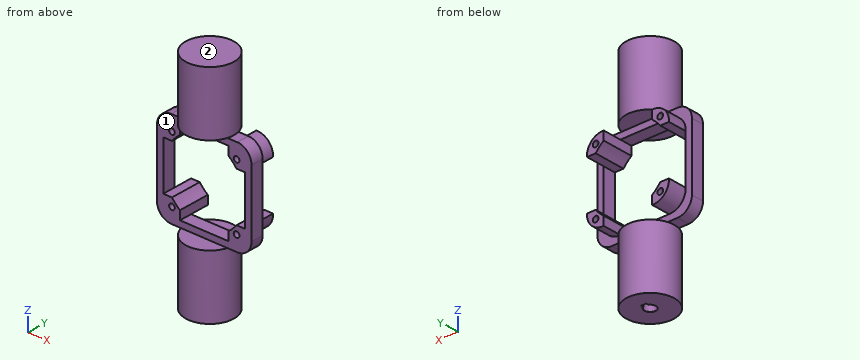
Autodesk Inventor part; units mm, degrees
ref_plane "YZ Plane" through (0, 0, 0) normal (1, 0, 0) x (0, 1, 0)
ref_plane "XZ Plane" through (0, 0, 0) normal (0, 1, 0) x (-1, 0, 0)
ref_plane "XY Plane" through (0, 0, 0) normal (0, 0, 1) x (1, 0, 0)
sketch "Sketch1" plane through (0, 0, 0) normal (0, 0, 1) x (1, 0, 0)
  circle A0 centre (0, 0) radius 38
  dimension "d0" = 76
extrude "Extrusion1" add sketch "Sketch1" along normal blind 100
sketch "Sketch2" plane through (0, 0, 0) normal (0, 0, -1) x (-1, 0, 0)
  circle A0 centre (0, 0) radius 8.75
  line L0 (0, 8.75) -> (0, 11.75)
  line L1 (0, 11.75) -> (4, 11.75)
  line L2 (4, 11.75) -> (-4, 11.75)
  line L3 (-4, 11.75) -> (-4, 7.7822)
  line L4 (4, 11.75) -> (4, 7.7822)
  dimension "d3" = 17.5
  dimension "d5" = 3
  dimension "d6" = 4
  dimension "d7" = 8
  dimension "d8" = 3.9678
  dimension "d9" = 3.9678
extrude "Extrusion2" cut sketch "Sketch2" against normal blind 90
fillet "Fillet1" radius 0.5 4 edges at (4, 9.7661, 0) (0, 11.75, 0) (-4, 9.7661, 0) (0, -8.75, 0)
fillet "Fillet2" radius 0.5 4 edges at (-4, 7.7822, 45.25) (-4.1498, 7.8731, 0.1431) (4, 7.7822, 45.25) (4.1498, 7.8731, 0.1431)
sketch "Sketch5" plane through (0, 0, 100) normal (0, 0, 1) x (1, 0, 0)
  line L0 (-75, -10) -> (75, -10)
  line L1 (75, -10) -> (75, 10)
  line L2 (75, 10) -> (-75, 10)
  line L3 (-75, 10) -> (-75, -10)
  line L4 (-75, -10) -> (75, 10) construction
  line L5 (75, -10) -> (-75, 10) construction
  point P0 (0, 0)
  dimension "d32" = 150
  dimension "d33" = 20
extrude "Extrusion5" add sketch "Sketch5" along normal blind 150
fillet "Fillet6" radius 22.751 4 edges at (-75, 0, 250) (75, 0, 250) (75, 0, 100) (-75, 0, 100)
sketch "Sketch8" plane through (0, 0, 250) normal (0, 0, 1) x (1, 0, 0)
  circle A0 centre (0, 0) radius 38
extrude "Extrusion8" add sketch "Sketch8" along normal blind 100
sketch "Sketch11" plane through (-36.6606, 10, 100) normal (0, 1, 0) x (1, 0, 0)
  line L0 (-28.3394, -140) -> (101.6606, -140)
  line L1 (101.6606, -140) -> (101.6606, -10)
  line L2 (101.6606, -10) -> (-28.3394, -10)
  line L3 (-28.3394, -10) -> (-28.3394, -140)
  line L4 (-28.3394, -140) -> (101.6606, -10) construction
  line L5 (101.6606, -140) -> (-28.3394, -10) construction
  line L6 (-38.3394, -22.751) -> (-38.3394, -127.249)
  line L7 (0, -150) -> (73.3212, -150)
  line L8 (-38.3394, -127.249) -> (-28.3394, -127.249)
  line L9 (-15.5884, -150) -> (0, -150)
  line L10 (-15.5884, -150) -> (-15.5884, -140)
  line L11 (-38.3394, -22.751) -> (-38.3394, -127.249)
  line L12 (-38.3394, -22.751) -> (-28.3394, -22.751)
  arc A0 (-15.5884, 0) -> (-38.3394, -22.751) centre (-15.5884, -22.751) ccw
  line L13 (-15.5884, 0) -> (-15.5884, -10)
  line L14 (88.9096, 0) -> (73.3212, 0)
  line L15 (88.9096, 0) -> (88.9096, -10)
  arc A1 (111.6606, -22.751) -> (88.9096, 0) centre (88.9096, -22.751) ccw
  line L16 (111.6606, -22.751) -> (101.6606, -22.751)
  line L17 (73.3212, -150) -> (88.9096, -150)
  line L18 (88.9096, -150) -> (88.9096, -140)
  line L19 (111.6606, -22.751) -> (111.6606, -127.249)
  line L20 (111.6606, -127.249) -> (101.6606, -127.249)
  line L21 (-28.3394, -75) -> (-28.3394, -36.5)
  line L22 (-28.3394, -75) -> (-28.3394, -113.5)
  line L23 (-28.3394, -36.5) -> (-14.5394, -36.5)
  line L24 (36.6606, -10) -> (-1.8394, -10)
  line L25 (36.6606, -10) -> (75.1606, -10)
  line L26 (-1.8394, -10) -> (-1.8394, -23.8)
  arc A2 (-1.8394, -23.8) -> (-14.5394, -36.5) centre (36.832, -75.1714) ccw
  line L27 (36.6606, -140) -> (-1.8394, -140)
  line L28 (36.6606, -140) -> (75.1606, -140)
  line L29 (101.6606, -75) -> (101.6606, -113.5)
  line L30 (101.6606, -75) -> (101.6606, -36.5)
  line L31 (36.6606, -10) -> (75.1606, -10)
  line L32 (-28.3394, -113.5) -> (-14.5394, -113.5)
  line L33 (-1.8394, -140) -> (-1.8394, -126.2)
  line L34 (75.1606, -140) -> (75.1606, -126.2)
  line L35 (101.6606, -113.5) -> (87.8606, -113.5)
  line L36 (101.6606, -36.5) -> (87.8606, -36.5)
  line L37 (75.1606, -10) -> (75.1606, -23.8)
  arc A3 (75.1606, -126.2) -> (87.8606, -113.5) centre (36.4892, -74.8286) ccw
  arc A4 (-14.5394, -113.5) -> (-1.8394, -126.2) centre (36.832, -74.8286) ccw
  arc A5 (87.8606, -36.5) -> (75.1606, -23.8) centre (36.4892, -75.1714) ccw
  point P0 (36.6606, 100)
  point P1 (36.6606, -75)
  dimension "d72" = 130
  dimension "d73" = 130
  dimension "d74" = 75
  dimension "d75" = 75
  dimension "d84" = 38.5
  dimension "d85" = 38.5
  dimension "d86" = 13.8
  dimension "d87" = 38.5
  dimension "d88" = 38.5
  dimension "d89" = 13.8
  dimension "d90" = 64.3
  dimension "d96" = 38.5
  dimension "d97" = 38.5
  dimension "d98" = 38.5
  dimension "d99" = 38.5
  dimension "d100" = 13.8
  dimension "d101" = 13.8
  dimension "d102" = 13.8
  dimension "d103" = 13.8
  dimension "d104" = 13.8
  dimension "d105" = 13.8
  dimension "d106" = 64.3
  dimension "d107" = 64.3
  dimension "d108" = 64.3
extrude "Extrusion10" cut sketch "Sketch11" against normal blind 20 contours L33 A4 L32 L3 L23 A2 L26 L2 L37 A5 L36 L1 L35 A3 L34 L0
sketch "Sketch12" plane through (-36.6606, 10, 100) normal (0, 1, 0) x (1, 0, 0)
  circle A0 centre (-14.6044, -23.735) radius 4.5
  line L0 (-28.3394, -36.5) -> (-14.5394, -36.5)
  line L1 (-28.3394, -113.5) -> (-28.3394, -36.5)
  circle A1 centre (-14.6044, -126.265) radius 4.5
  circle A2 centre (87.9256, -126.265) radius 4.5
  circle A3 centre (87.9256, -23.735) radius 4.5
  line L2 (-14.5394, -113.5) -> (-28.3394, -113.5)
  line L3 (101.6606, -113.5) -> (87.8606, -113.5)
  line L4 (101.6606, -36.5) -> (101.6606, -113.5)
  line L5 (87.8606, -36.5) -> (101.6606, -36.5)
  point P0 (36.6606, 100)
  point P1 (-28.3394, -127.249)
  dimension "d91" = 9
  dimension "d92" = 12.765
  dimension "d93" = 13.735
  dimension "d109" = 9
  dimension "d110" = 9
  dimension "d111" = 9
  dimension "d112" = 12.765
  dimension "d113" = 13.735
  dimension "d114" = 12.765
  dimension "d115" = 13.735
  dimension "d116" = 13.735
  dimension "d117" = 12.765
extrude "Extrusion11" cut sketch "Sketch12" along normal mid plane 50
sketch "Sketch13" plane through (-36.6606, 10, 100) normal (0, 1, 0) x (1, 0, 0)
  line L0 (-28.3394, -113.5) -> (-28.3394, -36.5)
  line L1 (75.1606, -140) -> (-1.8394, -140)
  arc A0 (-28.3394, -113.5) -> (-1.8394, -140) centre (-3.3874, -115.048) ccw
  line L2 (-1.8394, -10) -> (-1.8394, -23.8)
  arc A1 (-1.8394, -10) -> (-28.3394, -36.5) centre (-3.3874, -34.952) ccw
  line L3 (101.6606, -113.5) -> (101.6606, -36.5)
  arc A2 (75.1606, -140) -> (101.6606, -113.5) centre (76.7086, -115.048) ccw
  line L4 (101.6606, -36.5) -> (87.8606, -36.5)
  line L5 (75.1606, -23.8) -> (75.1606, -10)
  arc A3 (101.6606, -36.5) -> (75.1606, -10) centre (76.7086, -34.952) ccw
  line L6 (-1.8394, -126.2) -> (-1.8394, -140)
  line L7 (-1.8394, -140) -> (-1.8394, -126.2)
  arc A4 (-14.5394, -113.5) -> (-1.8394, -126.2) centre (36.832, -74.8286) ccw
  line L8 (-28.3394, -113.5) -> (-14.5394, -113.5)
  arc A5 (-14.5394, -113.5) -> (-1.8394, -126.2) centre (36.832, -74.8286) ccw
  line L9 (-14.5394, -36.5) -> (-28.3394, -36.5)
  line L10 (-28.3394, -36.5) -> (-14.5394, -36.5)
  line L11 (-1.8394, -10) -> (-1.8394, -23.8)
  line L12 (75.1606, -10) -> (75.1606, -23.8)
  line L13 (87.8606, -36.5) -> (101.6606, -36.5)
  line L14 (101.6606, -113.5) -> (87.8606, -113.5)
  line L15 (87.8606, -113.5) -> (101.6606, -113.5)
  arc A6 (-1.8394, -23.8) -> (-14.5394, -36.5) centre (36.832, -75.1714) ccw
  arc A7 (-1.8394, -23.8) -> (-14.5394, -36.5) centre (36.832, -75.1714) ccw
  arc A8 (87.8606, -36.5) -> (75.1606, -23.8) centre (36.4892, -75.1714) ccw
  line L16 (75.1606, -140) -> (75.1606, -126.2)
  line L17 (75.1606, -140) -> (75.1606, -126.2)
  arc A9 (75.1606, -126.2) -> (87.8606, -113.5) centre (36.4892, -74.8286) ccw
  arc A10 (75.1606, -126.2) -> (87.8606, -113.5) centre (36.4892, -74.8286) ccw
  point P0 (36.6606, 100)
  dimension "d118" = 25
  dimension "d119" = 25
  dimension "d120" = 25
  dimension "d121" = 25
  dimension "d122" = 64.3
  dimension "d125" = 64.3
  dimension "d126" = 64.3
  dimension "d127" = 64.3
extrude "Extrusion12" add sketch "Sketch13" along normal blind 30
sketch "Sketch14" plane through (-36.6606, -10, 100) normal (0, -1, 0) x (1, 0, 0)
  circle A0 centre (-14.6044, 23.735) radius 4.5
  circle A1 centre (-14.6044, 23.735) radius 4.5
  circle A2 centre (-14.6044, 126.265) radius 4.5
  circle A3 centre (-14.6044, 126.265) radius 4.5
  circle A4 centre (87.9256, 126.265) radius 4.5
  circle A5 centre (87.9256, 126.265) radius 4.5
  circle A6 centre (87.9256, 23.735) radius 4.5
  circle A7 centre (87.9256, 23.735) radius 4.5
  point P0 (36.6606, -100)
  dimension "d130" = 9
  dimension "d131" = 9
  dimension "d132" = 9
  dimension "d133" = 9
extrude "Extrusion13" cut sketch "Sketch14" against normal blind 100
equation "\"d112\" = d92"
equation "\"d113\" = d93"
equation "\"d114\" = d112"
equation "\"d115\" = d113"
equation "\"d116\" = d115"
equation "\"d117\" = d114"
properties part number "FrontPlateV2"
Part model, mm, in its own coordinate system. Face numbers are marked on the shaded views. A direction names the side the tool comes from. Round coordinates to 2 decimals unless told otherwise and drop trailing zeros. Write each loop counter-clockwise with the first axis right and the second up, starting at its lowest first coordinate (ties: lowest second). Pieces come first, ordered by that corner, then holes. Notation, with made-up numbers: (1.25, 31) - (36.25, 31) arc R9 ccw to (36.25, 40) - close; hole circle Ø5 at (59.5, 67.25). An arc over 180 degrees is marked (long way). Use CSV: the item, a comma, the result in double quotes.
Item 1: Slice it at C-C, the plane x = -22. Write the cut outline in (y, z), then the cut area to 3 significant figures.
Results list:
outline,"(-30.98, 0) - (30.98, 0) - (30.98, 100) - (10, 100) - (10, 110) - (-10, 110) - (-10, 100) - (-30.98, 100) - close; (-30.98, 250) - (-10, 250) - (-10, 240) - (10, 240) - (10, 250) - (30.98, 250) - (30.98, 350) - (-30.98, 350) - close"
area,"12,800 mm²"
Item 2: Flat gauge pins, fed straight in: P1, Ø12, axis at y = 12.5, z = 36, coming from the +X side; P2, Ø11, axis at x = 55, y = 16.5, coming from the -Z side; P3, Ø10, axis at y = 2.5, z = 87.5, coming from the +X side. Where does each tip first touch, or does it go through?
Results list:
P1,"stops at x = 37.44"
P2,"stops at z = 111.81"
P3,"stops at x = 38"
Item 3: Wall check: L1, parallel to Z at x = -9.5, y = 1; L2, parallel to X at y = -8.5, z = 144; L3, parallel to X at y = 7, z = 229. Give the ranges that are in metal, low to high.
Results list:
L1,"z = 0 to 110, 240 to 350"
L2,"x = -75 to -65, 65 to 75"
L3,"x = -74.93 to -54.84, -47.69 to -38.5, 38.5 to 47.69, 54.84 to 74.93"
Item 4: Tool access for the marked faces 1 and 2: list every direction of +Z, -Z, +X, -X, +Y, -Y with a clear straight run to the whole face (end or side of a thin tool).
Results list:
face 1,"+X, -X, -Y"
face 2,"+Z, +X, -X, +Y, -Y"
Item 5: Slice it at D-D, the plane z = 307. Write the cut outline in (x, y).
Results list:
outline,"circle Ø76 at (0, 0)"
Item 6: Slice it at B-B, the plane y = -17. Write the cut outline in (x, z), then the cut area to 3 significant figures.
Results list:
outline,"(-33.99, 0) - (33.99, 0) - (33.99, 100) - (-33.99, 100) - close; (-33.99, 250) - (33.99, 250) - (33.99, 350) - (-33.99, 350) - close"
area,"13,600 mm²"
Item 7: Slice it at A-A, the plane x = 0. Write the cut outline in (y, z).
Results list:
outline,"(-38, 0) - (-9.25, 0) arc R0.5 ccw to (-8.75, 0.5) - (-8.75, 90) - (11.75, 90) - (11.75, 0.5) arc R0.5 ccw to (12.25, 0) - (38, 0) - (38, 100) - (10, 100) - (10, 110) - (-10, 110) - (-10, 100) - (-38, 100) - close; (-38, 250) - (-10, 250) - (-10, 240) - (10, 240) - (10, 250) - (38, 250) - (38, 350) - (-38, 350) - close"
